```python
from build123d import *

# Parameters (mm, degrees)
F0_W           = 20
F0_H           = 3
F2_DEPTH       = 22.5
F3_D           = 13
F3_DEPTH       = 10
F3_TIP         = 3.9055940237
F4_D           = 22
F4_DEPTH       = 10
F4_TIP         = 6.6094668093
F7_D           = 10
F7_DEPTH       = 10
F7_TIP         = 3.0043030951
F7_ON_F5_D     = 10
F7_ON_F5_DEPTH = 10
F7_ON_F5_TIP   = 3.0043030951


# Not quite as in the source:
# - a feature names something its author has since deleted; it is built from what else it names


with BuildPart() as f2:
    # F0 (on Top) → F2 (new body, symmetric)
    with BuildSketch(Plane.XY):
        Polygon((-47, 0), (0, 0), (12, 0), (15, 0), (50, 0), (50, 3), (-50, 3), (-50, 0), align=None)
        Polygon((15, 0), (12, 0), (12, -60), (15, -60), (15, -57), align=None)
        Polygon((-47, -60), (-47, 0), (-50, 0), (-50, -57), (-50, -60), align=None)
        with Locations((-60, -58.5)):
            Rectangle(F0_W, F0_H)
        with Locations((25, -58.5)):
            Rectangle(F0_W, F0_H)
    extrude(amount=F2_DEPTH, both=True)

    # F3 (one way)
    with BuildSketch(Plane.XZ):
        with Locations((32.5, 0)):
            Circle(F3_D / 2)
    extrude(amount=-F3_DEPTH, mode=Mode.SUBTRACT)
    with Locations(Plane.XZ):
        with Locations((32.5, 0)):
            with Locations((0, 0, -(F3_DEPTH + F3_TIP / 2))):  # 118° drill point
                Cone(0, F3_D / 2, F3_TIP, mode=Mode.SUBTRACT)

    # F4
    with Locations(Plane.XZ):
        with Locations((-17.5, 0)):
            Hole(F4_D / 2, depth=F4_DEPTH)
            with Locations((0, 0, -(F4_DEPTH + F4_TIP / 2))):  # 118° drill point
                Cone(0, F4_D / 2, F4_TIP, mode=Mode.SUBTRACT)

    # F7 (one way)
    with BuildSketch(Plane(origin=(0, -57, 0), x_dir=(-1, 0, 0), z_dir=(0, 1, 0))):
        with Locations((-25, 0)):
            Circle(F7_D / 2)
    extrude(amount=-F7_DEPTH, mode=Mode.SUBTRACT)
    with Locations(Plane(origin=(0, -57, 0), x_dir=(-1, 0, 0), z_dir=(0, 1, 0))):
        with Locations((-25, 0)):
            with Locations((0, 0, -(F7_DEPTH + F7_TIP / 2))):  # 118° drill point
                Cone(0, F7_D / 2, F7_TIP, mode=Mode.SUBTRACT)

    # F7 on F5
    with Locations(Plane(origin=(0, -57, 0), x_dir=(-1, 0, 0), z_dir=(0, 1, 0))):
        with Locations((60, 0)):
            Hole(F7_ON_F5_D / 2, depth=F7_ON_F5_DEPTH)
            with Locations((0, 0, -(F7_ON_F5_DEPTH + F7_ON_F5_TIP / 2))):  # 118° drill point
                Cone(0, F7_ON_F5_D / 2, F7_ON_F5_TIP, mode=Mode.SUBTRACT)


solid = f2.part
```
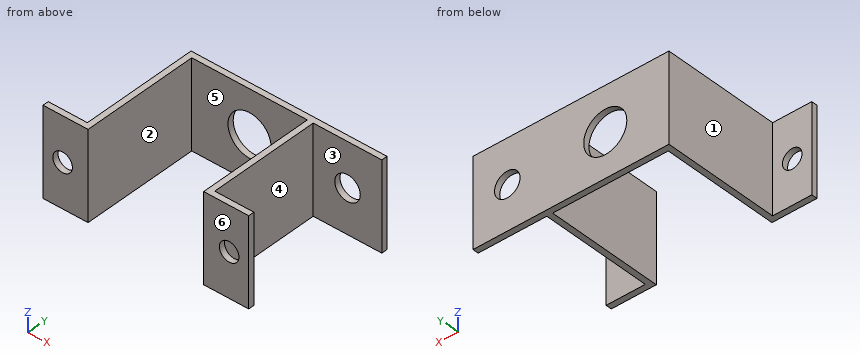
Geometry: final body of the model. Coordinates: model frame, mm. Face numbers are marked on the shaded views. A direction names the side the tool comes from. Round coordinates to 2 decimals unless told otherwise and drop trailing zeros. Write each loop counter-clockwise with the first axis right and the second up, starting at its lowest first coordinate (ties: lowest second). Pieces come first, ordered by that corner, then holes. Notation, with made-up numbers: (-9, 45.5) -> (38, 45.5) arc R23 ccw to (38, 62.5) -> close; hole circle Ø6 at (48, -15.75). An arc over 180 degrees is marked (long way). Use CSV: the item, a comma, the result in double quotes. Start each with the question number.
Q1. Pull-direction query (X, two-part tool) for the marked faces 4, 5 and 6; classes: pulls with the +X half, pulls with the -X half, needs draft (parallel to the pull), parting line crosses it, or undercut.
Q2. Section D-D (x = 32.5). Return loops of the section in (y, z), plus the area to 3 significant figures.
Q3. Section A-A (z = 0). Give the number of separate pieces and of enclosed holes in the cut face, plus the area to 3 significant figures.
Q4. Section C-C (y = -17). Return loops of the section in (x, z), plus the area to 3 significant figures.
Q5. Line query: L1, parallel to X at y = -20, z = -5.5; L2, parallel to Z at x = -17, y = 2; L3, parallel to Z at x = 25, y = -59. Output: solid intervals per line, ascending.
Q6. Section B-B (x = -60). Return loops of the section in (y, z), plus the area to 3 significant figures.
Q7. First-contact query: pin 1 Ø13.5 at (x, z) = (-7, 3.5) entering from -Y; pin 2 Ø8 at (x, y) = (-40, -7.5) entering from -Z; pin 3 Ø3 at (y, z) = (-36.5, -8.5) entering from +X; pin 4 Ø6 at (x, z) = (-60.5, -10.5) entering from +Y. Flat tips, straight axial feed; report the tip coordinate or a pass-through.
Q8. Reachability of the marked faces 1, 2 and 3 from +Z, -Z, +X, -X, +Y, -Y: full face, straight path, thin tool, end or side. Return the list, or none.
Result sheet:
1,face 4,"pulls with the +X half"
1,face 5,"undercut"
1,face 6,"needs draft"
2,outline,"(-60, -22.5) -> (-57, -22.5) -> (-57, 22.5) -> (-60, 22.5) -> close; (0, -22.5) -> (3, -22.5) -> (3, -6.5) -> (0, -6.5) -> close; (0, 6.5) -> (3, 6.5) -> (3, 22.5) -> (0, 22.5) -> close"
2,area,"231 mm²"
3,separate pieces,"5"
3,enclosed holes,"0"
3,area,"615 mm²"
4,outline,"(-50, -22.5) -> (-47, -22.5) -> (-47, 22.5) -> (-50, 22.5) -> close; (12, -22.5) -> (15, -22.5) -> (15, 22.5) -> (12, 22.5) -> close"
4,area,"270 mm²"
5,L1,"-50 to -47, 12 to 15"
5,L2,"-22.5 to -10.99, 10.99 to 22.5"
5,L3,"-22.5 to -5, 5 to 22.5"
6,outline,"(-60, -22.5) -> (-57, -22.5) -> (-57, -5) -> (-60, -5) -> close; (-60, 5) -> (-57, 5) -> (-57, 22.5) -> (-60, 22.5) -> close"
6,area,"105 mm²"
7,pin 1,"y = 0"
7,pin 2,"through"
7,pin 3,"x = 15"
7,pin 4,"y = -57"
8,face 1,"+Z, -Z, -X, +Y"
8,face 2,"+Z, -Z, -Y"
8,face 3,"+Z, -Z, +X"
